Could you check a few things on this model? Use its own coordinates, in mm. Face numbers are marked on the shaded views. Coordinates: 2 decimals unless noted, no trailing zeros. Order: outer loops, then holes, each group sorted by start corner. A loop starts at its lowest first (then second) coordinate and runs counter-clockwise, first axis right, second up. Notation, with made-up numbers: (87.25, 24.25) - (117.25, 24.25) arc R13 ccw to (117.25, 45.25) - close; hole circle Ø8 at (23, 30). An arc over 180 degrees is marked (long way). One line per item, written item: value. Start each with the question number.
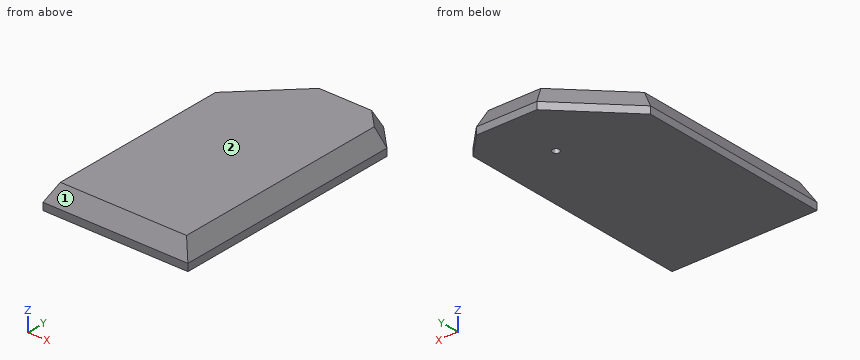
from build123d import *

# Parameters (mm, degrees)
BOSS_EXTRUDE1_DEPTH           = 7
BOSS_EXTRUDE1_TAPER           = 29
BOSS_EXTRUDE1_OTHER_WAY_DEPTH = 3
SKETCH2_R                     = 1.5
CUT_EXTRUDE1_DEPTH            = 3


with BuildPart() as part:
    # Sketch1 → Boss-Extrude1 (new body)
    with BuildSketch(Plane.XY):
        Polygon((-57.811201834, -26.002477708), (2.188798166, -26.002477708), (2.188798166, 70.629617347), (-7.398088721, 80.216504233), (-32.398088721, 80.216504233), (-57.811201834, 54.80339112), align=None)
    extrude(amount=BOSS_EXTRUDE1_DEPTH, taper=BOSS_EXTRUDE1_TAPER)

    # Sketch1 → Boss-Extrude1 other way (add)
    with BuildSketch(Plane.XY):
        Polygon((-57.811201834, -26.002477708), (2.188798166, -26.002477708), (2.188798166, 70.629617347), (-7.398088721, 80.216504233), (-32.398088721, 80.216504233), (-57.811201834, 54.80339112), align=None)
    extrude(amount=-BOSS_EXTRUDE1_OTHER_WAY_DEPTH)

    # Sketch2 → Cut-Extrude1 (cut)
    with BuildSketch(Plane(origin=(0, 0, -3), x_dir=(-1, 0, 0), z_dir=(0, 0, -1))):
        with Locations((19.898088721, 56.224723903)):
            Circle(SKETCH2_R)
    extrude(amount=-CUT_EXTRUDE1_DEPTH, mode=Mode.SUBTRACT)


solid = part.part
Q1. If I drill on L1, parallel to X at y = 7.5, z = 1; L2, parallel to Y at x = -29, z = 1.75; L3, parallel to X at y = -8, z = 6.25, over which ranges is the centre line in solid material (lowest first)?
Q2. I want a section at A-A on z = -1.25. Please give me the cut outline in (x, y).
Q3. I want a section at C-C on x = -15. Please give me the cut outline in (y, z).
Q4. I'm going to push flat-ended pins straight in: pin 1 (6 mm diameter, centred on x = -36.5, z = -1.5, fed in from +Y); pin 2 (4 mm diameter, centred on y = 6, z = 2.5, fed in from -X). Where does each tip first touch, or does it pass through?
Q5. I want a section at B-B on y = -3. Please give me the cut outline in (x, z).
Q6. We'd pull the mould along Y, two halves only. Please class the marked faces 1 and 2: +Y half, -Y half, draft (parallel to the pull), parting line (faces both ways), or undercut.
Values follow:
1. L1: x = -57.26 to 1.63
1. L2: y = -25.03 to 79.25
1. L3: x = -54.35 to -1.28
2. outline: (-57.81, -26) - (2.19, -26) - (2.19, 70.63) - (-7.4, 80.22) - (-32.4, 80.22) - (-57.81, 54.8) - close; hole circle Ø3 at (-19.9, 56.22)
3. outline: (-26, -3) - (80.22, -3) - (80.22, 0) - (76.34, 7) - (-22.12, 7) - (-26, 0) - close
4. pin 1: stops at y = 79.11
4. pin 2: stops at x = -57.53
5. outline: (-57.81, -3) - (2.19, -3) - (2.19, 0) - (-1.69, 7) - (-53.93, 7) - (-57.81, 0) - close
6. face 1: -Y half
6. face 2: draft
